Here's the drawing with two shaded views (mm, measured from the low corner). I have some questions. A direction names the side the tool comes from. Coordinates: 2 decimals unless noted, no trailing zeros. Order: outer loops, then holes, each group sorted by start corner. A loop starts at its lowest first (then second) coordinate and runs counter-clockwise, first axis right, second up. Notation, with made-up numbers: M 27.5,-21.75 L 65.5,-21.75 A30 cw 65.5,1.25 Z; hole C 55,59.25 d8. An arc over 180 degrees is marked long. Put each result on its own line as item: value. Start each with the question number.
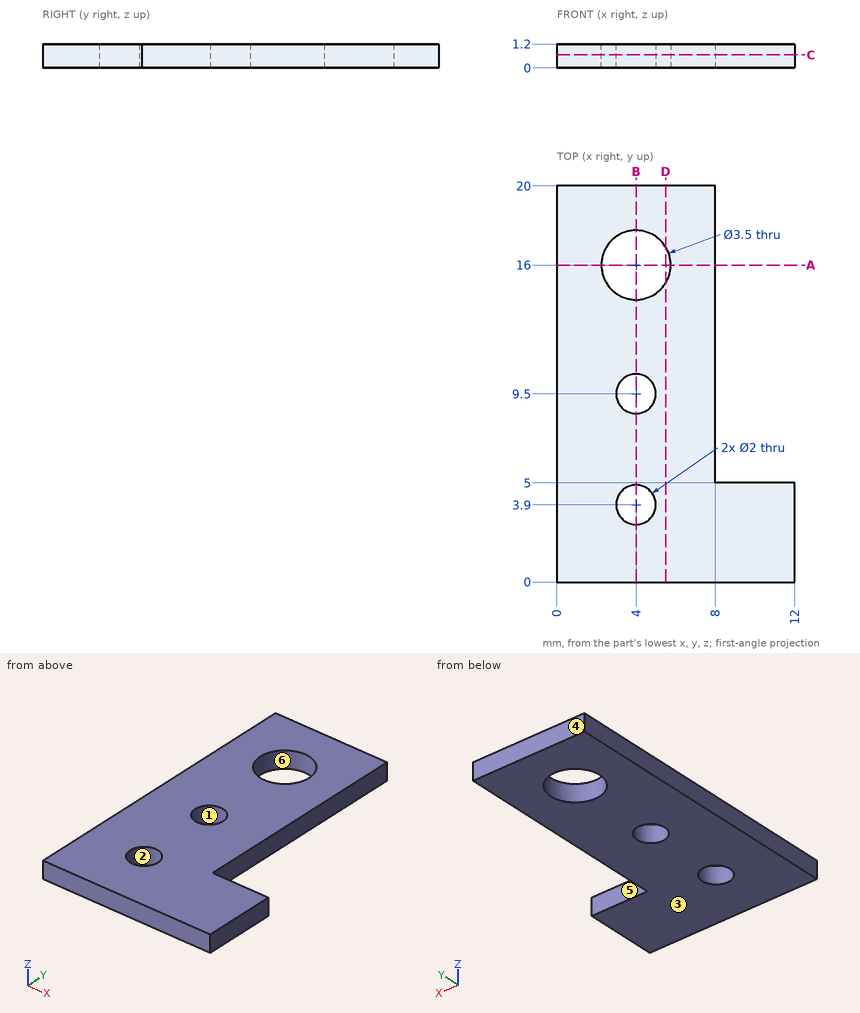
Item 1: For the marked faces 5 and 6, which set-ups out of +Z, -Z, +X, -X, +Y, -Y let a thin tool reach every point of the face, with its end or its side?
Item 2: For pin 1 Ø3 at (x, y) = (4, 16) entering from -Z, with a flat end and sliding along its axis, tell me the tip position at first contact or that it passes through.
Item 3: I need wall thicknesses on probe 1 along Y at (x, z) = (4, 0.8); probe 2 along Y at (x, z) = (4.75, 0.8); probe 3 along X at (y, z) = (12, 0.1). Which ranges of each line are inside material? Lowest first, please.
Item 4: If we section it at C-C on z = 0.65: Write out the boundary of the cut face in (x, y), then the cut area to 3 significant figures.
Item 5: If we section it at B-B on x = 4: Write out the boundary of the cut face in (y, z).
Item 6: If we section it at A-A on y = 16: Write out the boundary of the cut face in (x, z), then the cut area to 3 significant figures.
Item 7: If we section it at D-D on x = 5.5: Write out the boundary of the cut face in (y, z).
Item 8: If we mould it in two halves opening along Y, with no side actions, what happens to the marked faces 1, 2, 3 and 4? For each: released by +Y, released by -Y, zero draft, split by the parting line, or undercut.
Geometry check:
1. face 5: +Z, -Z, +X, +Y
1. face 6: +Z, -Z
2. pin 1: passes through
3. probe 1: y = 0 to 2.9, 4.9 to 8.5, 10.5 to 14.25, 17.75 to 20
3. probe 2: y = 0 to 3.24, 4.56 to 8.84, 10.16 to 14.42, 17.58 to 20
3. probe 3: x = 0 to 8
4. outline: M 0,0 L 12,0 L 12,5 L 8,5 L 8,20 L 0,20 Z; hole C 4,16 d3.5; hole C 4,3.9 d2; hole C 4,9.5 d2
4. area: 164 mm²
5. outline: M 0,0 L 2.9,0 L 2.9,1.2 L 0,1.2 Z; M 4.9,0 L 8.5,0 L 8.5,1.2 L 4.9,1.2 Z; M 10.5,0 L 14.25,0 L 14.25,1.2 L 10.5,1.2 Z; M 17.75,0 L 20,0 L 20,1.2 L 17.75,1.2 Z
6. outline: M 0,0 L 2.25,0 L 2.25,1.2 L 0,1.2 Z; M 5.75,0 L 8,0 L 8,1.2 L 5.75,1.2 Z
6. area: 5.40 mm²
7. outline: M 0,0 L 15.1,0 L 15.1,1.2 L 0,1.2 Z; M 16.9,0 L 20,0 L 20,1.2 L 16.9,1.2 Z
8. face 1: undercut
8. face 2: undercut
8. face 3: zero draft
8. face 4: released by +Y
